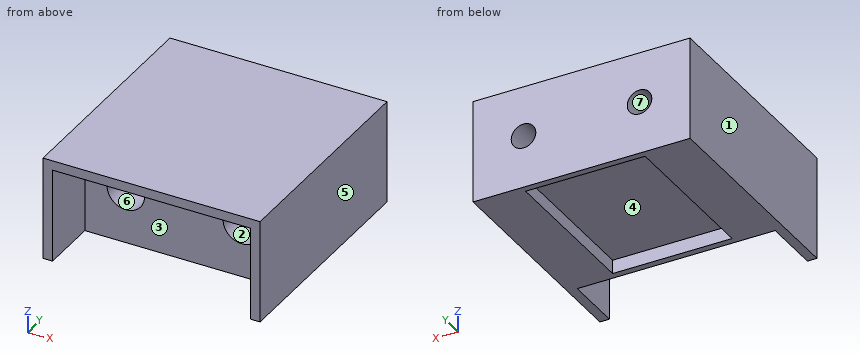
from build123d import *

# Parameters (mm, degrees)
SKETCH004_W     = 31.8
SKETCH004_H     = 33.4
PAD002_DEPTH    = 15.1
SKETCH005_W     = 29.000001
SKETCH005_H     = 13.7
POCKET001_DEPTH = 8.5
SKETCH006_W     = 17.5
SKETCH006_H     = 22.9
POCKET002_DEPTH = 2
SKETCH009_R     = 2.75
POCKET004_DEPTH = 8
SKETCH010_R     = 1.8
POCKET005_DEPTH = 20


with BuildPart() as part:
    # Sketch004 (on Face5 of Binder001) → Pad002 (new body)
    with BuildSketch(Plane.XY.offset(1.6)):
        with Locations((13.749781, 17.25)):
            Rectangle(SKETCH004_W, SKETCH004_H)
    extrude(amount=PAD002_DEPTH)

    # Sketch005 (on Face2 of Pad002) → Pocket001 (cut)
    with BuildSketch(Plane.XZ.offset(-0.55)):
        with Locations((13.74978, 8.45)):
            Rectangle(SKETCH005_W, SKETCH005_H)
    extrude(amount=-POCKET001_DEPTH, mode=Mode.SUBTRACT)

    # Sketch006 (on Face4 of Pocket001) → Pocket002 (cut)
    with BuildSketch(Plane(origin=(0, 0, 1.6), x_dir=(1, 0, 0), z_dir=(0, 0, -1))):
        with Locations((13.75, -21.5)):
            Rectangle(SKETCH006_W, SKETCH006_H)
    extrude(amount=-POCKET002_DEPTH, mode=Mode.SUBTRACT)

    # Sketch009 (on Face10 of Pocket002) → Pocket004 (cut)
    with BuildSketch(Plane.XZ.offset(-9.05)):
        with Locations((5.24978, 9.3)):
            Circle(SKETCH009_R)
        with Locations((22.249781, 9.3)):
            Circle(SKETCH009_R)
    extrude(amount=-POCKET004_DEPTH, mode=Mode.SUBTRACT)

    # Sketch010 (on Face18 of Pocket004) → Pocket005 (cut)
    with BuildSketch(Plane.XZ.offset(-17.05)):
        with Locations((5.24978, 9.3)):
            Circle(SKETCH010_R)
        with Locations((22.249781, 9.3)):
            Circle(SKETCH010_R)
    extrude(amount=-POCKET005_DEPTH, mode=Mode.SUBTRACT)


solid = part.part
For this review, take the finished solid that the model builds, in its own axes (mm). Face numbers are marked on the shaded views. A direction names the side the tool comes from. Coordinates: 2 decimals unless noted, no trailing zeros. Order: outer loops, then holes, each group sorted by start corner. A loop starts at its lowest first (then second) coordinate and runs counter-clockwise, first axis right, second up. Notation, with made-up numbers: (58, 3.25) - (115, 3.25) arc R22 cw to (115, 17.25) - close; hole circle Ø8 at (-32.5, -25.75). An arc over 180 degrees is marked (long way). Answer as CSV lines item,"result". Start each with the question number.
1) Add section D-D (x = 4). State the section outline as (y, z) points, then the cut area to 3 significant figures.
2) Draft analysis for pull direction Z (two halves, no side actions). For the marked faces 4, 5, 6 and 7, state which applies: +Z half, -Z half, draft (parallel to the pull), parting line (faces both ways), or undercut.
3) To check wall thickness, follow line 1 along X through (y, z) = (2.5, 8); line 2 along X through (y, z) = (27, 9.5); line 3 along Y through (x, z) = (21.5, 15.25). State the ranges of each line that lie inside material, in increasing order. Write a range as [from, to].
4) Add section C-C (z = 5.5). State the section outline as (x, y) points.
5) Add section A-A (z = 9.3). State the section outline as (x, y) points.
6) Add section B-B (y = 29). State the section outline as (x, z) points, then the cut area to 3 significant figures.
7) Machinability: for the marked faces 1, 2 and 3, which of the approach directions +Z, -Z, +X, -X, +Y, -Y give a long, thin tool a straight path to every point of the face, cutting with its end or side? Answer none if there is none.
8) Insertion check: P1, Ø2.5, axis at x = 18, y = 6, coming from the -Z side; P2, Ø9, axis at x = 13, y = 20.5, coming from the -Z side; P3, Ø6, axis at x = 4, z = 10, coming from the -Y side. Each pin has a flat end and moves straight along its axis. Give the tip position at first contact, or say it passes through.
Result:
1,outline,"(0.55, 15.3) - (9.05, 15.3) - (9.05, 11.75) - (17.05, 11.75) - (17.05, 10.6) - (33.95, 10.6) - (33.95, 16.7) - (0.55, 16.7) - close; (9.05, 1.6) - (33.95, 1.6) - (33.95, 8) - (17.05, 8) - (17.05, 6.85) - (9.05, 6.85) - close"
1,area,"305 mm^2"
2,face 4,"-Z half"
2,face 5,"draft"
2,face 6,"undercut"
2,face 7,"undercut"
3,line 1,"[-2.15, -0.75], [28.25, 29.65]"
3,line 2,"[-2.15, 3.46], [7.04, 20.46], [24.04, 29.65]"
3,line 3,"[9.05, 33.95]"
4,outline,"(-2.15, 0.55) - (-0.75, 0.55) - (-0.75, 9.05) - (28.25, 9.05) - (28.25, 0.55) - (29.65, 0.55) - (29.65, 33.95) - (-2.15, 33.95) - close"
5,outline,"(-2.15, 0.55) - (-0.75, 0.55) - (-0.75, 9.05) - (2.5, 9.05) - (2.5, 17.05) - (3.45, 17.05) - (3.45, 33.95) - (-2.15, 33.95) - close; (7.05, 17.05) - (8, 17.05) - (8, 9.05) - (19.5, 9.05) - (19.5, 17.05) - (20.45, 17.05) - (20.45, 33.95) - (7.05, 33.95) - close; (24.05, 17.05) - (25, 17.05) - (25, 9.05) - (28.25, 9.05) - (28.25, 0.55) - (29.65, 0.55) - (29.65, 33.95) - (24.05, 33.95) - close"
6,outline,"(-2.15, 1.6) - (5, 1.6) - (5, 3.6) - (22.5, 3.6) - (22.5, 1.6) - (29.65, 1.6) - (29.65, 16.7) - (-2.15, 16.7) - close; hole circle Ø3.6 at (5.25, 9.3); hole circle Ø3.6 at (22.25, 9.3)"
6,area,"425 mm^2"
7,face 1,"+Z, -Z, -X, +Y, -Y"
7,face 2,"-Y"
7,face 3,"-Z, -Y"
8,P1,"z = 15.3"
8,P2,"z = 3.6"
8,P3,"y = 9.05"
